```python
from build123d import *

# Parameters (mm, degrees)
F1_DEPTH = 3.25


# Not quite as in the source:
# - a feature names something its author has since deleted; it is built from what else it names


with BuildPart() as f1:
    # F0 (on Top) → F1 (new body)
    with BuildSketch(Plane.XY):
        with BuildLine():
            Line((-15.0887755982, 9.6346731841), (-18.5, 9.6346731841))
            Line((-18.5, 9.6346731841), (-18.5, -10.3653268159))
            Line((-18.5, -10.3653268159), (-15.0627288748, -10.3653268159))
            ThreePointArc((-15.0627288748, -10.3653268159), (-14.2270313471, -10.1144637876), (-13.719482936, -10.824194178))
            ThreePointArc((-13.719482936, -10.824194178), (-13.7932388225, -11.1485302676), (-14, -11.4090751683))
            Line((-14, -11.4090751683), (-14, -15))
            Line((-14, -15), (14, -15))
            Line((14, -15), (14, -11.3693879251))
            ThreePointArc((14, -11.3693879251), (13.9880219466, -10.2502281458), (15.1013118376, -10.3653268159))
            Line((15.1013118376, -10.3653268159), (18.5, -10.3653268159))
            Line((18.5, -10.3653268159), (18.5, 9.6346731841))
            Line((18.5, 9.6346731841), (15.021365697, 9.6376556492))
            ThreePointArc((15.021365697, 9.6376556492), (13.9052912015, 9.611890406), (14, 10.7242376408))
            Line((14, 10.7242376408), (14, 15))
            Line((14, 15), (-14, 15))
            Line((-14, 15), (-14, 10.6527720123))
            ThreePointArc((-14, 10.6527720123), (-13.8060615496, 10.3964917422), (-13.7372004166, 10.082565248))
            ThreePointArc((-13.7372004166, 10.082565248), (-14.251278169, 9.3706377987), (-15.0887755982, 9.6346731841))
        make_face()
    extrude(amount=F1_DEPTH)


solid = f1.part
```
Part model, mm, in its own coordinate system. A direction names the side the tool comes from. Give positions to 0.01 mm unless a question says otherwise; leave off trailing zeros. Order: outer loops, then holes, each group sorted by start corner. A loop starts at its lowest first (then second) coordinate and runs counter-clockwise, first axis right, second up. Notation, with made-up numbers: M 42.25,-5 L 97.25,-5 A29 ccw 97.25,22 Z; hole C 21.25,12.25 d3. An arc over 180 degrees is marked long. Use a Markdown table: item, result. Add a question column.
(1) 3-axis set-ups, long thin cutter, end or side, ignore diameter. For faces 5 (the face through (-17, 9.635, 2)), 6 (the face through (17, -10.365, 2)), 7 (the face through (-17, -10.365, 2)): which of +Z, -Z, +X, -X, +Y, -Y reach the whole face in a straight line?
(2) Mould opens along Y. For faces 1 (the face through (13.918, 9.599, 1.602)), 2 (the face through (0, 15, 2)), 3 (the face through (13.98, -10.26, 1.6)), 4 (the face through (14, 13, 2)) say: +Y half, -Y half, draft (parallel to the pull), parting line (faces both ways), or undercut.
(3) Probe line 1 along Y through (x, z) = (16, 0.9); line 2 along X through (y, z) = (11, 1.85); line 3 along Y through (x, z) = (-15, 0.45). List the from-to ranges inside material, lowest first. Write a range as [from, to].
(4) Saw through at A-A, the plane z = 1. Give the cut face in (x, y).
(5) Saw through at B-B, the plane x = 16. Give the cut face in (y, z), and give its area (3 significant figures).
(6) Drop flat-ended pins along their axis: P1, Ø1.6, axis at x = -17.5, z = 2, coming from the -Y side; P2, Ø1.3, axis at x = 14.45, y = 10.13, coming from the -Z side. Give the stop position or say it passes through.
Answer key:
| question | item | result |
|---|---|---|
| 1 | face 5 | +Z, -Z, -X, +Y |
| 1 | face 6 | +Z, -Z, +X, -Y |
| 1 | face 7 | +Z, -Z, -X, -Y |
| 2 | face 1 | undercut |
| 2 | face 2 | +Y half |
| 2 | face 3 | undercut |
| 2 | face 4 | draft |
| 3 | line 1 | [-10.37, 9.64] |
| 3 | line 2 | [-14, 14] |
| 3 | line 3 | [-10.29, 9.54] |
| 4 | outline | M -18.5,-10.37 L -15.06,-10.37 A0.75 cw long -14,-11.41 L -14,-15 L 14,-15 L 14,-11.37 A0.75 cw long 15.1,-10.37 L 18.5,-10.37 L 18.5,9.63 L 15.02,9.64 A0.75 cw long 14,10.72 L 14,15 L -14,15 L -14,10.65 A0.75 cw long -15.09,9.63 L -18.5,9.63 Z |
| 5 | outline | M -10.37,0 L 9.64,0 L 9.64,3.25 L -10.37,3.25 Z |
| 5 | area | 65.0 mm^2 |
| 6 | P1 | y = -10.37 |
| 6 | P2 | through |
